Check sheet for the drawn part. Datum: minimum x, y, z corner. Units: mm. A direction names the side the tool comes from. Give positions to 0.01 mm unless a question says otherwise; leave off trailing zeros. Write each loop counter-clockwise with the first axis right and the second up, starting at its lowest first coordinate (ties: lowest second). Pieces come first, ordered by that corner, then holes. Notation, with made-up numbers: (45.5, 62) - (50.5, 62) arc R22 ccw to (50.5, 69) - close; hole circle Ø11 at (-27, 57). An arc over 180 degrees is marked (long way). Use a Markdown table: item, result.
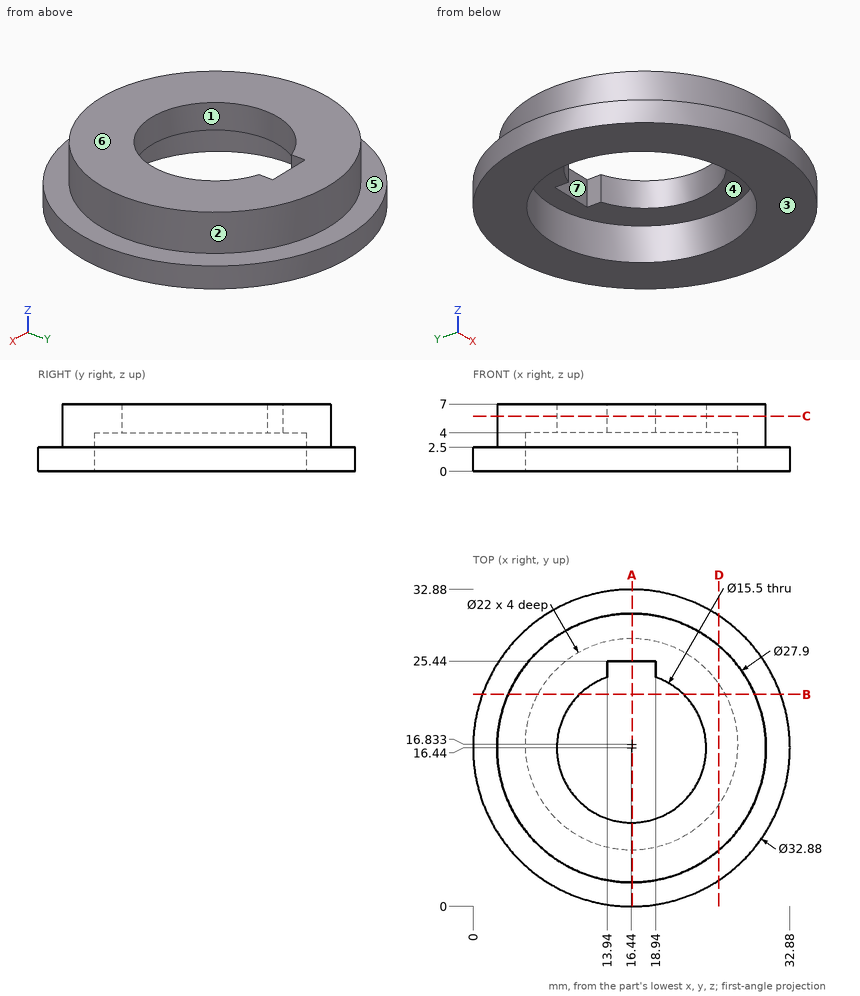
1) Set-up check for the marked faces 4, 5, 6 and 7: record each of +Z, -Z, +X, -X, +Y, -Y from which the full face is reachable in a straight line by a thin tool's end or side.
Working result:
| item | result |
|---|---|
| face 4 | -Z |
| face 5 | +Z |
| face 6 | +Z, +X, -X, +Y, -Y |
| face 7 | +Z, -Z |
2) Material ranges on L1, parallel to Z at x = 14.5, y = 26; L2, parallel to Z at x = 5.5, y = 26; L3, parallel to Y at x = 17, z = 1.75, recorded low to high. Write a range as from..to.
Working result:
| item | result |
|---|---|
| L1 | z = 4..7 |
| L2 | z = 0..2.5 |
| L3 | y = 0.01..5.85, 27.82..32.87 |
3) Mould release check, pull along Y, two halves, no side actions. Record for the marked faces 1, 2 and 3: pulls with the +Y half, pulls with the -Y half, needs draft (parallel to the pull), parting line crosses it, or undercut.
Working result:
| item | result |
|---|---|
| face 1 | undercut |
| face 2 | parting line crosses it |
| face 3 | needs draft |
4) Section check C-C on z = 5.75. Record the boundary of the cut face in (x, y).
Working result:
| item | result |
|---|---|
| outline | circle Ø27.9 at (16.44, 16.44); hole (13.94, 23.78) arc R7.75 ccw (long way) to (18.94, 23.78) - (18.94, 25.44) - (13.94, 25.44) - close |
5) Section check D-D on x = 25.5. Record the boundary of the cut face in (y, z) (1 decimal), then the cut area to 3 significant figures.
Working result:
| item | result |
|---|---|
| outline | (2.7, 0) - (10.6, 0) - (10.6, 4) - (23.1, 4) - (23.1, 0) - (30.2, 0) - (30.2, 2.5) - (27, 2.5) - (27, 7) - (5.8, 7) - (5.8, 2.5) - (2.7, 2.5) - close |
| area | 114 mm² |
6) Depth check by flat-ended pin: P1, Ø1.5, axis at y = 19.5, z = 3, coming from the -X side; P2, Ø17.5, axis at x = 16.5, y = 18, coming from the -Z side; P3, Ø0.8, axis at y = 24, z = 5, coming from the -X side. Enter the tip coordinate at first touch or a pass-through.
Working result:
| item | result |
|---|---|
| P1 | stops at x = 0.19 |
| P2 | stops at z = 4 |
| P3 | stops at x = 4.47 |
7) Section check B-B on y = 22. Record the boundary of the cut face in (x, z) (1 decimal).
Working result:
| item | result |
|---|---|
| outline | (1, 0) - (6.7, 0) - (6.7, 4) - (11, 4) - (11, 7) - (3.6, 7) - (3.6, 2.5) - (1, 2.5) - close; (21.8, 4) - (26.2, 4) - (26.2, 0) - (31.9, 0) - (31.9, 2.5) - (29.2, 2.5) - (29.2, 7) - (21.8, 7) - close |
8) Section check A-A on x = 16.5. Record the boundary of the cut face in (y, z).
Working result:
| item | result |
|---|---|
| outline | (0, 0) - (5.83, 0) - (5.83, 4) - (8.69, 4) - (8.69, 7) - (2.49, 7) - (2.49, 2.5) - (0, 2.5) - close; (25.44, 4) - (27.83, 4) - (27.83, 0) - (32.88, 0) - (32.88, 2.5) - (30.39, 2.5) - (30.39, 7) - (25.44, 7) - close |
